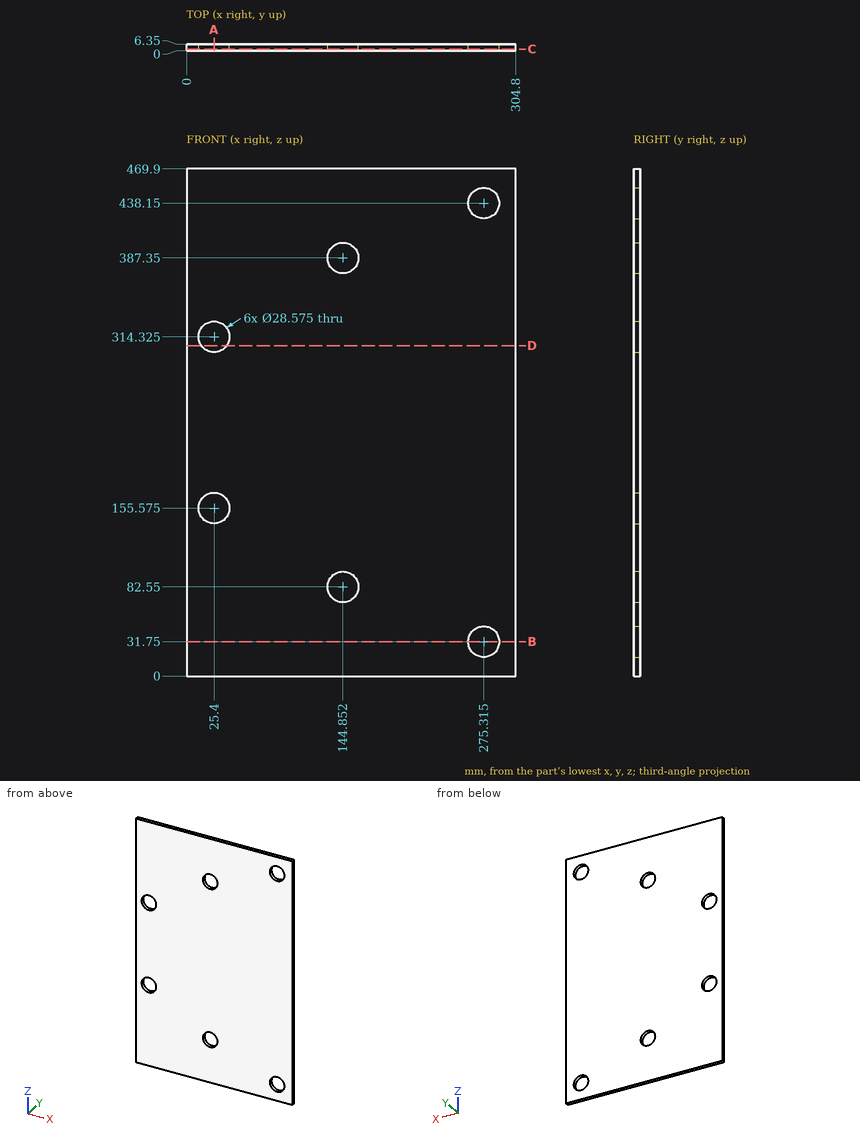
Could you check a few things on this drawing? It's one solid part, dimensions in mm from its lowest x, y, z. Coordinates: 2 decimals unless noted, no trailing zeros. Write each loop counter-clockwise with the first axis right and the second up, starting at its lowest first coordinate (ties: lowest second). Pieces come first, ordered by that corner, then holes. Notation, with made-up numbers: (-6.5, -32) - (18.5, -32) arc R10 ccw to (18.5, -20) - close; hole circle Ø7 at (22, 64.25). An arc over 180 degrees is marked (long way). Return JSON: item names as keys, results as strings. Group by question number.
Item 1: If we section it at A-A (x = 25.4): Write out the boundary of the cut face in (y, z), then the cut area to 3 significant figures.
Item 2: Please list where these lines run through material, in increasing order: probe 1 along X at (y, z) = (3.25, 82.55); probe 2 along X at (y, z) = (5.5, 439); probe 3 along Z at (x, y) = (263, 3.75) (1 decimal).
Item 3: I'm going to push flat-ended pins straight in: pin 1 Ø3 at (x, z) = (96.5, 56) entering from -Y; pin 2 Ø23 at (x, z) = (25.4, 314.325) entering from +Y. Where does each tip first touch, or does it pass through?
Item 4: If we section it at B-B (z = 31.75): Write out the boundary of the cut face in (x, y).
Item 5: If we section it at D-D (z = 306): Write out the boundary of the cut face in (x, y), then the cut area to 3 significant figures.
Item 6: If we section it at C-C (y = 1.5): Count the separate pieces of the cut face and the enclosed holes in it, then the cut area to 3 significant figures.
Return value:
{
 "1": {"outline": "(0, 0) - (6.35, 0) - (6.35, 141.29) - (0, 141.29) - close; (0, 169.86) - (6.35, 169.86) - (6.35, 300.04) - (0, 300.04) - close; (0, 328.61) - (6.35, 328.61) - (6.35, 469.9) - (0, 469.9) - close", "area": "2,620 mm^2"},
 "2": {"probe 1": "x = 0 to 130.56, 159.14 to 304.8", "probe 2": "x = 0 to 261.05, 289.58 to 304.8", "probe 3": "z = 0 to 24.5, 39 to 430.9, 445.4 to 469.9"},
 "3": {"pin 1": "stops at y = 0", "pin 2": "passes through"},
 "4": {"outline": "(0, 0) - (261.03, 0) - (261.03, 6.35) - (0, 6.35) - close; (289.6, 0) - (304.8, 0) - (304.8, 6.35) - (289.6, 6.35) - close"},
 "5": {"outline": "(0, 0) - (13.79, 0) - (13.79, 6.35) - (0, 6.35) - close; (37.01, 0) - (304.8, 0) - (304.8, 6.35) - (37.01, 6.35) - close", "area": "1,790 mm^2"},
 "6": {"separate pieces": "1", "enclosed holes": "6", "area": "139,000 mm^2"}
}
